Could you check a few things on this model? Use its own coordinates, in mm. A direction names the side the tool comes from. Give positions to 0.01 mm unless a question says otherwise; leave off trailing zeros. Loops run counter-clockwise (first coordinate to the right, second up) from the corner with the lowest first, then second, coordinate; pieces in that order, holes last.
1. Imagine slicing it at D-D (x = 12). List the corners of the cut face in (y, z) for me.
2. Imagine slicing it at B-B (z = 0). List the corners of the cut face in (x, y) for me (3 decimals), plus the area to 3 significant figures.
3. I need wall thicknesses on line 1 along X through (y, z) = (2.15, 0) (3 decimals); line 2 along X through (y, z) = (11, 0) (3 decimals). Which ranges of each line are inside material? Lowest first, please.
4. For faces 1 (the cylindrical face through (10.902, 2.576, -3.433)), 2 (the flat face through (4, 5.08, 11)), which set-ups out of +Z, -Z, +X, -X, +Y, -Y let a thin tool reach every point of the face, with its end or its side?
5. For P1, Ø3, axis at x = -4, z = 10.5, coming from the +Y side; P2, Ø2, axis at x = -8, z = -4, coming from the -Y side; P3, Ø2, axis at y = 5, z = 8, coming from the -X side; P4, Ø4, axis at x = -2.5, y = 2, coming from the +Z side, each with a flat end and sliding along its axis, tell me the tip position at first contact or that it passes through.
6. Imagine slicing it at C-C (y = 7). List the corners of the cut face in (x, z) for me (3 decimals), plus the area to 3 significant figures.
7. Imagine slicing it at A-A (x = 0). List the corners of the cut face in (y, z) for me (3 decimals).
```python
from build123d import *

# Parameters (mm, degrees)
SKETCH1_R               = 18.415
BOSS_EXTRUDE1_DEPTH     = 12.7
SKETCH2_R               = 16.891
CUT_EXTRUDE1_DEPTH      = 7.62
SKETCH3_R               = 11.43
CUT_EXTRUDE2_DEPTH      = 8.62
CUT_EXTRUDE2_DEPTH_BACK = 6.08


with BuildPart() as part:
    # Sketch1 → Boss-Extrude1 (new body)
    with BuildSketch(Plane(origin=(0, 0, 0), x_dir=(1, 0, 0), z_dir=(0, 1, 0))):
        Circle(SKETCH1_R)
    extrude(amount=BOSS_EXTRUDE1_DEPTH)

    # Sketch2 → Cut-Extrude1 (cut)
    with BuildSketch(Plane(origin=(0, 12.7, 0), x_dir=(1, 0, 0), z_dir=(0, 1, 0))):
        Circle(SKETCH2_R)
    extrude(amount=-CUT_EXTRUDE1_DEPTH, mode=Mode.SUBTRACT)

    # Sketch3 → Cut-Extrude2 (cut, two sides)
    with BuildSketch(Plane(origin=(0, 5.08, 0), x_dir=(1, 0, 0), z_dir=(0, 1, 0))) as cut_extrude2_sk:
        Circle(SKETCH3_R)
    extrude(amount=CUT_EXTRUDE2_DEPTH, mode=Mode.SUBTRACT)
    extrude(cut_extrude2_sk.sketch, amount=-CUT_EXTRUDE2_DEPTH_BACK, mode=Mode.SUBTRACT)


solid = part.part
```
Derived:
1. outline: (0, -13.97) - (12.7, -13.97) - (12.7, -11.89) - (5.08, -11.89) - (5.08, 11.89) - (12.7, 11.89) - (12.7, 13.97) - (0, 13.97) - close
2. outline: (-18.415, 0) - (-11.43, 0) - (-11.43, 5.08) - (-16.891, 5.08) - (-16.891, 12.7) - (-18.415, 12.7) - close; (11.43, 0) - (18.415, 0) - (18.415, 12.7) - (16.891, 12.7) - (16.891, 5.08) - (11.43, 5.08) - close
2. area: 94.2 mm2
3. line 1: x = -18.415 to -11.43, 11.43 to 18.415
3. line 2: x = -18.415 to -16.891, 16.891 to 18.415
4. face 1: +Y, -Y
4. face 2: +Y
5. P1: stops at y = 5.08
5. P2: passes through
5. P3: stops at x = -17.03
5. P4: stops at z = 18.41
6. outline: circle Ø36.83 at (0, 0); hole circle Ø33.782 at (0, 0)
6. area: 169 mm2
7. outline: (0, -18.415) - (12.7, -18.415) - (12.7, -16.891) - (5.08, -16.891) - (5.08, -11.43) - (0, -11.43) - close; (0, 11.43) - (5.08, 11.43) - (5.08, 16.891) - (12.7, 16.891) - (12.7, 18.415) - (0, 18.415) - close
